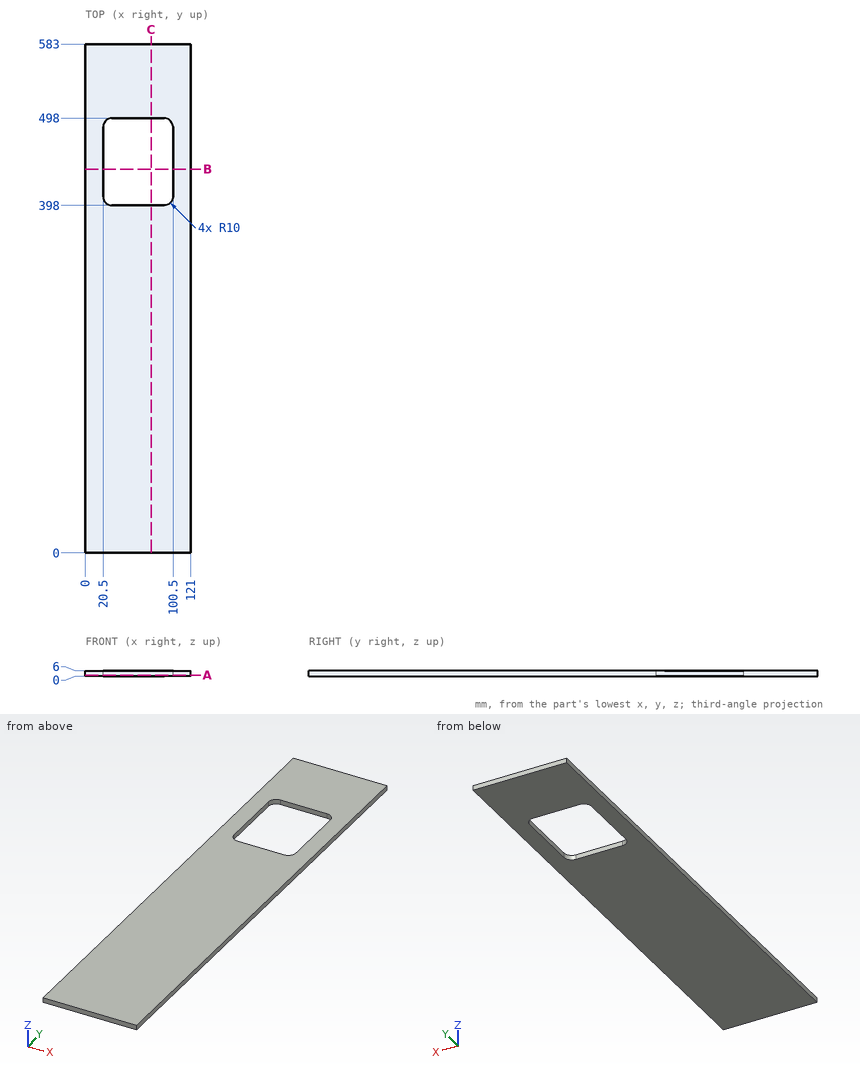
Study the drawing (mm; zero at the part's minimum x, y, z) and answer. Give positions to 0.01 mm unless a question says otherwise; leave off trailing zeros. Write each loop counter-clockwise with the first axis right and the second up, starting at its lowest first coordinate (ties: lowest second). Pieces come first, ordered by that corner, then holes. Notation, with made-up numbers: (-38.5, 77.5) - (20.5, 77.5) arc R18 ccw to (20.5, 89.5) - close; hole circle Ø1 at (58, -18). An arc over 180 degrees is marked (long way). Write item = value, one per line. Start each with the question number.
Item 1: Find section A-A (z = 0.95). Give the vertices of the cut face in (x, y), then the cut area to 3 significant figures.
Item 2: Find section B-B (y = 439.5). Give the vertices of the cut face in (x, z), then the cut area to 3 significant figures.
Item 3: Find the intervals of material crossed by probe 1 along Y at (x, z) = (65.5, 5.1); probe 2 along Y at (x, z) = (91.5, 0.25); probe 3 along X at (y, z) = (413, 1.2), in increasing order. Write a range as [from, to].
Item 4: Find section C-C (x = 75.5). Give the vertices of the cut face in (y, z).
Response:
q1.outline = (0, 0) - (121, 0) - (121, 583) - (0, 583) - close; hole (20.5, 408) arc R10 ccw to (30.5, 398) - (90.5, 398) arc R10 ccw to (100.5, 408) - (100.5, 488) arc R10 ccw to (90.5, 498) - (30.5, 498) arc R10 ccw to (20.5, 488) - close
q1.area = 62,600 mm²
q2.outline = (0, 0) - (20.5, 0) - (20.5, 6) - (0, 6) - close; (100.5, 0) - (121, 0) - (121, 6) - (100.5, 6) - close
q2.area = 246 mm²
q3.probe_1 = [0, 398], [498, 583]
q3.probe_2 = [0, 398.05], [497.95, 583]
q3.probe_3 = [0, 20.5], [100.5, 121]
q4.outline = (0, 0) - (398, 0) - (398, 6) - (0, 6) - close; (498, 0) - (583, 0) - (583, 6) - (498, 6) - close
